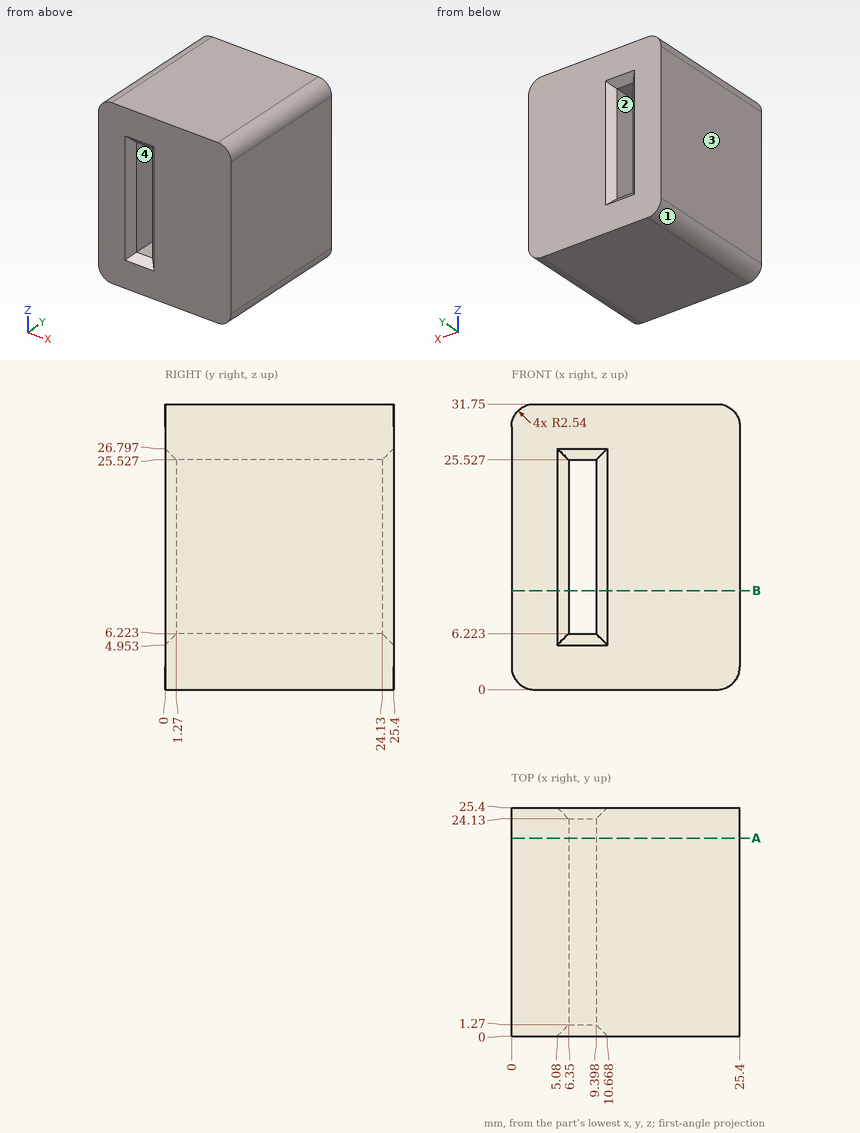
For this review, use the dimensioned drawing (mm, ordinates from the lowest corner) and the shaded views. Give positions to 0.01 mm unless a question says otherwise; leave off trailing zeros. Loops run counter-clockwise (first coordinate to the right, second up) from the corner with the lowest first, then second, coordinate; pieces in that order, holes last.
Item 1: Insertion check: pin 1 (1 mm diameter, centred on x = 6, z = 17, fed in from -Y). The pin has a flat end and moves straight along its axis. Give the tip position at first contact, or say it passes through.
Item 2: Take a section at A-A, the plane y = 22. State the section outline as (x, z) points, and give its area (3 significant figures).
Item 3: Draft analysis for pull direction Z (two halves, no side actions). For the marked faces 1, 2, 3 and 4, state which applies: +Z half, -Z half, draft (parallel to the pull), parting line (faces both ways), or undercut.
Item 4: For line 1 along X through (y, z) = (11.75, 22); line 2 along Z through (x, y) = (8, 21.75), list the stretches that pass through material, from the lowest coordinate up.
Item 5: Take a section at B-B, the plane z = 11. State the section outline as (x, y) points, and give its area (3 significant figures).
Calculated:
1. pin 1: stops at y = 0.42
2. outline: (0, 2.54) arc R2.54 ccw to (2.54, 0) - (22.86, 0) arc R2.54 ccw to (25.4, 2.54) - (25.4, 29.21) arc R2.54 ccw to (22.86, 31.75) - (2.54, 31.75) arc R2.54 ccw to (0, 29.21) - close; hole (6.35, 6.22) - (9.4, 6.22) - (9.4, 25.53) - (6.35, 25.53) - close
2. area: 742 mm2
3. face 1: -Z half
3. face 2: undercut
3. face 3: draft
3. face 4: undercut
4. line 1: x = 0 to 6.35, 9.4 to 25.4
4. line 2: z = 0 to 6.22, 25.53 to 31.75
5. outline: (0, 0) - (5.08, 0) - (6.35, 1.27) - (6.35, 24.13) - (5.08, 25.4) - (0, 25.4) - close; (9.4, 1.27) - (10.67, 0) - (25.4, 0) - (25.4, 25.4) - (10.67, 25.4) - (9.4, 24.13) - close
5. area: 565 mm2
